Verification items for the finished model (mm, model axes). Round coordinates to 2 decimals unless told otherwise and drop trailing zeros. Loops run counter-clockwise (first coordinate to the right, second up) from the corner with the lowest first, then second, coordinate; pieces in that order, holes last. Notation, with made-up numbers: (72.5, 19.25) - (98.5, 19.25) arc R21 cw to (98.5, 48.25) - close; hole circle Ø4 at (-22, 84). An arc over 180 degrees is marked (long way). Use a Markdown table: item, result. Add a question column.
```python
from build123d import *

# Parameters (mm, degrees)
F1_DEPTH = 2.9718
F2_R     = 1.651
F2_W     = 12.7
F2_H     = 25.4
F3_DEPTH = 2.9728


with BuildPart() as f1:
    # F0 (on Top) → F1 (new body)
    with BuildSketch(Plane.XY):
        Polygon((0, 152.4), (0, 0), (76.2, 0), (76.2, 152.4), (82.55, 152.4), (82.55, 222.25), (76.2, 222.25), (0, 222.25), (-6.35, 222.25), (-6.35, 152.4), align=None)
    extrude(amount=F1_DEPTH)

    # F2 (on face) → F3 (cut, through all)
    with BuildSketch(Plane.XY.offset(2.9718)):
        with Locations((38.1, 215.9)):
            Circle(F2_R)
        with Locations((60.96, 184.15)):
            Circle(F2_R)
        with Locations((15.24, 184.15)):
            Circle(F2_R)
        with Locations((38.1, 184.15)):
            Rectangle(F2_W, F2_H)
        Polygon((34.29, 6.35), (34.29, 0), (41.91, 0), (41.91, 6.35), (48.26, 6.35), (48.26, 4.318), (52.07, 4.318), (52.07, 6.35), (57.15, 6.35), (57.15, 9.652), (52.07, 9.652), (52.07, 11.684), (48.26, 11.684), (48.26, 9.652), (41.91, 9.652), (41.91, 50.8), (34.29, 50.8), (34.29, 9.652), (27.94, 9.652), (27.94, 11.684), (24.13, 11.684), (24.13, 9.652), (19.05, 9.652), (19.05, 6.35), (24.13, 6.35), (24.13, 4.318), (27.94, 4.318), (27.94, 6.35), align=None)
        with Locations((101.6, 63.5)):
            Circle(F2_R)
        Polygon((-3.302, 176.275976), (-6.35, 176.275976), (-6.35, 167.893976), (-3.302, 167.893976), (-3.302, 170.433976), (1.778, 170.433976), (1.778, 168.401976), (5.588, 168.401976), (5.588, 170.433976), (8.636, 170.433976), (8.636, 173.735976), (5.588, 173.735976), (5.588, 175.767976), (1.778, 175.767976), (1.778, 173.735976), (-3.302, 173.735976), align=None)
        Polygon((-3.302002, 207.009976), (-6.350002, 207.009976), (-6.350002, 198.627976), (-3.302002, 198.627976), (-3.302002, 201.167976), (1.777998, 201.167976), (1.777998, 199.135976), (5.587998, 199.135976), (5.587998, 201.167976), (8.635998, 201.167976), (8.635998, 204.469976), (5.587998, 204.469976), (5.587998, 206.501976), (1.777998, 206.501976), (1.777998, 204.469976), (-3.302002, 204.469976), align=None)
        Polygon((79.502, 198.627971), (82.55, 198.627971), (82.55, 207.009971), (79.502, 207.009971), (79.502, 204.469971), (74.422, 204.469971), (74.422, 206.501971), (70.612, 206.501971), (70.612, 204.469971), (67.564, 204.469971), (67.564, 201.167971), (70.612, 201.167971), (70.612, 199.135971), (74.422, 199.135971), (74.422, 201.167971), (79.502, 201.167971), align=None)
        Polygon((79.502002, 167.893971), (82.550002, 167.893971), (82.550002, 176.275971), (79.502002, 176.275971), (79.502002, 173.735971), (74.422002, 173.735971), (74.422002, 175.767971), (70.612002, 175.767971), (70.612002, 173.735971), (67.564002, 173.735971), (67.564002, 170.433971), (70.612002, 170.433971), (70.612002, 168.401971), (74.422002, 168.401971), (74.422002, 170.433971), (79.502002, 170.433971), align=None)
        with Locations((38.1, 139.7)):
            Circle(F2_R)
    extrude(amount=-F3_DEPTH, mode=Mode.SUBTRACT)


solid = f1.part
```
Q1. Thickness scan on line 1 along Y through (x, z) = (38.1, 1.65); line 2 along X through (y, z) = (184.15, 1.6); line 3 along Y through (x, z) = (55, 1.55). Record the ranges inside material, lowest first.
Q2. Go/stop test with flat-tipped pins: pin 1 Ø1.5 at (y, z) = (172.5, 1.5) entering from -X; pin 2 Ø1 at (y, z) = (205, 1.5) entering from +X; pin 3 Ø0.9 at (x, z) = (73, 2) entering from -Y; pin 4 Ø1 at (y, z) = (5.5, 1.5) entering from +X. Record where each tip stops, or that it passes through.
Q3. Section check A-A on y = 24. Record the cut outline in (x, z), plus the area to 3 significant figures.
Q4. Section check B-B on z = 1.5. State how many separate pieces and enclosed holes the cut face has, plus the area to 3 significant figures.
Determined:
| question | item | result |
|---|---|---|
| 1 | line 1 | y = 50.8 to 138.05, 141.35 to 171.45, 196.85 to 214.25, 217.55 to 222.25 |
| 1 | line 2 | x = -6.35 to 13.59, 16.89 to 31.75, 44.45 to 59.31, 62.61 to 82.55 |
| 1 | line 3 | y = 0 to 6.35, 9.65 to 222.25 |
| 2 | pin 1 | stops at x = 8.64 |
| 2 | pin 2 | stops at x = 79.5 |
| 2 | pin 3 | stops at y = 0 |
| 2 | pin 4 | stops at x = 76.2 |
| 3 | outline | (0, 0) - (34.29, 0) - (34.29, 2.97) - (0, 2.97) - close; (41.91, 0) - (76.2, 0) - (76.2, 2.97) - (41.91, 2.97) - close |
| 3 | area | 204 mm² |
| 4 | separate pieces | 1 |
| 4 | enclosed holes | 5 |
| 4 | area | 16,600 mm² |
